Source: CAD feature listing. Evaluate the final solid. Frame: model axes, mm. A direction names the side the tool comes from. Coordinates: 2 decimals unless noted, no trailing zeros. Order: outer loops, then holes, each group sorted by start corner. A loop starts at its lowest first (then second) coordinate and runs counter-clockwise, first axis right, second up. Notation, with made-up numbers: (-5, 3.5) - (45, 3.5) arc R12 cw to (45, 12.5) - close; hole circle Ø7 at (80, 66.5). An arc over 180 degrees is marked (long way). One line per question, with ' | ' between items.
from build123d import *

# Parameters (mm, degrees)
BOSS_EXTRUDE1_DEPTH     = 20
BOSS_EXTRUDE2_DEPTH     = 20
CUT_EXTRUDE3_DEPTH      = 29.776552955
CUT_EXTRUDE3_DEPTH_BACK = 29.776552955
CUT_EXTRUDE4_DEPTH      = 29.776552955
BOSS_EXTRUDE3_DEPTH     = 3
CUT_EXTRUDE5_DEPTH      = 29.776552955
SKETCH11_R              = 2
CUT_EXTRUDE6_DEPTH      = 25.98179337
SKETCH12_R              = 2
CUT_EXTRUDE7_DEPTH      = 10


with BuildPart() as part:
    # Sketch1 → Boss-Extrude1 (new body)
    with BuildSketch(Plane.XY):
        Polygon((-3, 6), (3, 6), (3, 4.1), (5.3, 4.1), (5.3, 2.48), (2.8, 0), (-2.8, 0), (-5.3, 2.48), (-5.3, 4.1), (-3, 4.1), align=None)
    extrude(amount=BOSS_EXTRUDE1_DEPTH)

    # Sketch2 → Boss-Extrude2 (add)
    with BuildSketch(Plane(origin=(-0.009718496, 0, -0.066979448), x_dir=(-1, 0, 0), z_dir=(0, 1, 0))):
        Polygon((-3.009718496, 6.066979448), (2.990281504, 6.066979448), (2.990281504, 4.166979448), (5.290281504, 4.166979448), (5.290281504, 2.546979448), (2.790281504, 0.066979448), (-2.809718496, 0.066979448), (-5.309718496, 2.546979448), (-5.309718496, 4.166979448), (-3.009718496, 4.166979448), align=None)
    extrude(amount=BOSS_EXTRUDE2_DEPTH)

    # Sketch3 → Cut-Extrude3 (cut, two sides: drawn at the far end of the back side and taken through both)
    with BuildSketch(Plane(origin=(0, 0, 0), x_dir=(1, 0, 0), z_dir=(0, 1, 0)).offset(-CUT_EXTRUDE3_DEPTH_BACK)):
        Polygon((-2.8, 0), (-5.3, -2.48), (-5.3, 0), align=None)
        Polygon((5.3, -2.48), (5.3, 0), (2.8, 0), align=None)
    extrude(amount=CUT_EXTRUDE3_DEPTH + CUT_EXTRUDE3_DEPTH_BACK, mode=Mode.SUBTRACT)

    # Sketch4 → Cut-Extrude4 (cut, through all)
    with BuildSketch(Plane.XY):
        Polygon((2.8, 0), (3, 0), (5.3, 0), (5.3, 2.48), align=None)
        Polygon((-5.3, 2.48), (-5.3, 0), (-3, 0), (-2.8, 0), align=None)
    extrude(amount=CUT_EXTRUDE4_DEPTH, mode=Mode.SUBTRACT)

    # Sketch5 → Boss-Extrude3 (add, symmetric)
    with BuildSketch(Plane(origin=(0, 0, 0), x_dir=(0, 0, -1), z_dir=(1, 0, 0))):
        Polygon((-11.656854249, 6), (-6, 6), (-6, 11.656854249), align=None)
    extrude(amount=BOSS_EXTRUDE3_DEPTH, both=True)

    # Sketch10 → Cut-Extrude5 (cut, through all)
    with BuildSketch(Plane(origin=(0, 0, 0), x_dir=(1, 0, 0), z_dir=(0, 1, 0))):
        Polygon((-5.3, -4.1), (-3, -4.1), (-3, -6), (-3, -6.6), (-5.3, -6.6), align=None)
        Polygon((3, -6), (3, -4.1), (5.3, -4.1), (5.3, -6.6), (3, -6.6), align=None)
    extrude(amount=CUT_EXTRUDE5_DEPTH, mode=Mode.SUBTRACT)

    # Sketch11 → Cut-Extrude6 (cut, through all)
    with BuildSketch(Plane.XY.offset(6)):
        with Locations((0, 16)):
            Circle(SKETCH11_R)
    extrude(amount=-CUT_EXTRUDE6_DEPTH, mode=Mode.SUBTRACT)

    # Sketch12 → Cut-Extrude7 (cut)
    with BuildSketch(Plane(origin=(0, 6, 0), x_dir=(1, 0, 0), z_dir=(0, 1, 0))):
        with Locations(Location((0, -16, 0), (0, 0, 270))):
            Circle(SKETCH12_R)
    extrude(amount=-CUT_EXTRUDE7_DEPTH, mode=Mode.SUBTRACT)


solid = part.part
(1) Set-up query: faces 1 (the flat face through (-4, 3, 6.6)), 2 (the flat face through (1, 14, 6)), 3 (the flat face through (4, 4.1, 13)), 4 (the flat face through (-4, 4.1, 13)). Return all of +Z, -Z, +X, -X, +Y, -Y with unobstructed straight access to the full face (end or side cutting, diameter ignored); none if empty.
Taken from the geometry:
face 1: -X, +Y, -Y | face 2: +Z, +X, -X, +Y | face 3: +Z, +X, +Y | face 4: +Z, -X, +Y
(2) Cut plane B-B (x = 0). Return the cut outline in (y, z), and give its area (3 significant figures).
Taken from the geometry:
outline: (0, 0) - (14, 0) - (14, 6) - (11.66, 6) - (6, 11.66) - (6, 14) - (0, 14) - close; (0, 18) - (6, 18) - (6, 20) - (0, 20) - close; (18, 0) - (20, 0) - (20, 6) - (18, 6) - close | area: 172 mm²
(3) Cut plane A-A (y = 16). Return the cut outline in (x, z), and give its area (3 significant figures).
Taken from the geometry:
outline: (-5.3, 2.48) - (-2.8, 0) - (-2, 0) - (-2, 6) - (-3, 6) - (-3, 4.1) - (-5.3, 4.1) - close; (2, 0) - (2.8, 0) - (5.3, 2.48) - (5.3, 4.1) - (3, 4.1) - (3, 6) - (2, 6) - close | area: 24.7 mm²
(4) Cut plane D-D (z = 4.75). Return the cut outline in (x, y), and give its area (3 significant figures).
Taken from the geometry:
outline: (-3, 0.2) - (-2.8, 0) - (2.8, 0) - (3, 0.2) - (3, 20) - (-3, 20) - close; hole circle Ø4 at (0, 16) | area: 107 mm²
(5) Material intervals for L1, parallel to X at y = 4.4, z = 16; L2, parallel to Y at x = 0, z = 4.5; L3, parallel to Z at x = 1.25, y = 12.75, sorted ascending. Write a range as from..to.
Taken from the geometry:
L1: x = -3..-2, 2..3 | L2: y = 0..14, 18..20 | L3: z = 0..6
(6) Pin query (flat end, axial travel): P1, Ø1.2, axis at x = 4.5, y = 1.5, coming from the -Z side; P2, Ø2.5, axis at x = 4, y = 15, coming from the +Z side; P3, Ø5, axis at x = -1, z = 11.5, coming from the +Y side. Return the tip coordinate at first contact, or that it passes through.
Taken from the geometry:
P1: stops at z = 1.09 | P2: stops at z = 6 | P3: stops at y = 8.66
(7) Pull-direction query (Y, two-part tool) for faces 5 (the flat face through (0, 20, 3)), 6 (the cylindrical face through (-1.774, 3.042, 16.923)), 7 (the cylindrical face through (0, 18, 3)); classes: pulls with the +Y half, pulls with the -Y half, needs draft (parallel to the pull), parting line crosses it, or undercut.
Taken from the geometry:
face 5: pulls with the +Y half | face 6: needs draft | face 7: undercut
